Geometry: see drawing. Coordinates: mm, zero at the bounding-box minimum. A direction names the side the tool comes from. Round coordinates to 2 decimals unless told otherwise and drop trailing zeros. Write each loop counter-clockwise with the first axis right and the second up, starting at its lowest first coordinate (ties: lowest second). Pieces come first, ordered by that corner, then holes. Notation, with made-up numbers: M 18.25,73 L 63.25,73 A14 cw 63.25,86 Z; hole C -21,3 d11. An arc over 180 degrees is marked long. Use one line per item in the form item = value. Start each with the question number.
Item 1: Pull-direction query (X, two-part tool) for the marked faces 3, 4 and 5; classes: pulls with the +X half, pulls with the -X half, needs draft (parallel to the pull), parting line crosses it, or undercut.
Item 2: Section query C-C (y = 14.75). Return loops of the section in (x, z), and give its area (3 significant figures).
Item 3: Section query D-D (x = 19.5). Return loops of the section in (y, z), and give its area (3 significant figures).
Item 4: Section query A-A (x = 32.5). Return loops of the section in (y, z), and give its area (3 significant figures).
Item 5: Pin query (flat end, axial travel): pin 1 Ø8 at (y, z) = (13, 27) entering from -X. Return the tip coordinate at first contact, or that it passes through.
Item 6: Reachability of the marked faces 1 and 2 from +Z, -Z, +X, -X, +Y, -Y: full face, straight path, thin tool, end or side. Return the list, or none.
Item 7: Section query B-B (z = 50). Return loops of the section in (x, y).
Item 8: Ray query, probe 1 along Z at (x, y) = (32.5, 29.35); probe 2 along X at (y, z) = (28.6, 50); probe 3 along X at (y, z) = (25, 75.5). Return the intervals inside material, ascending.
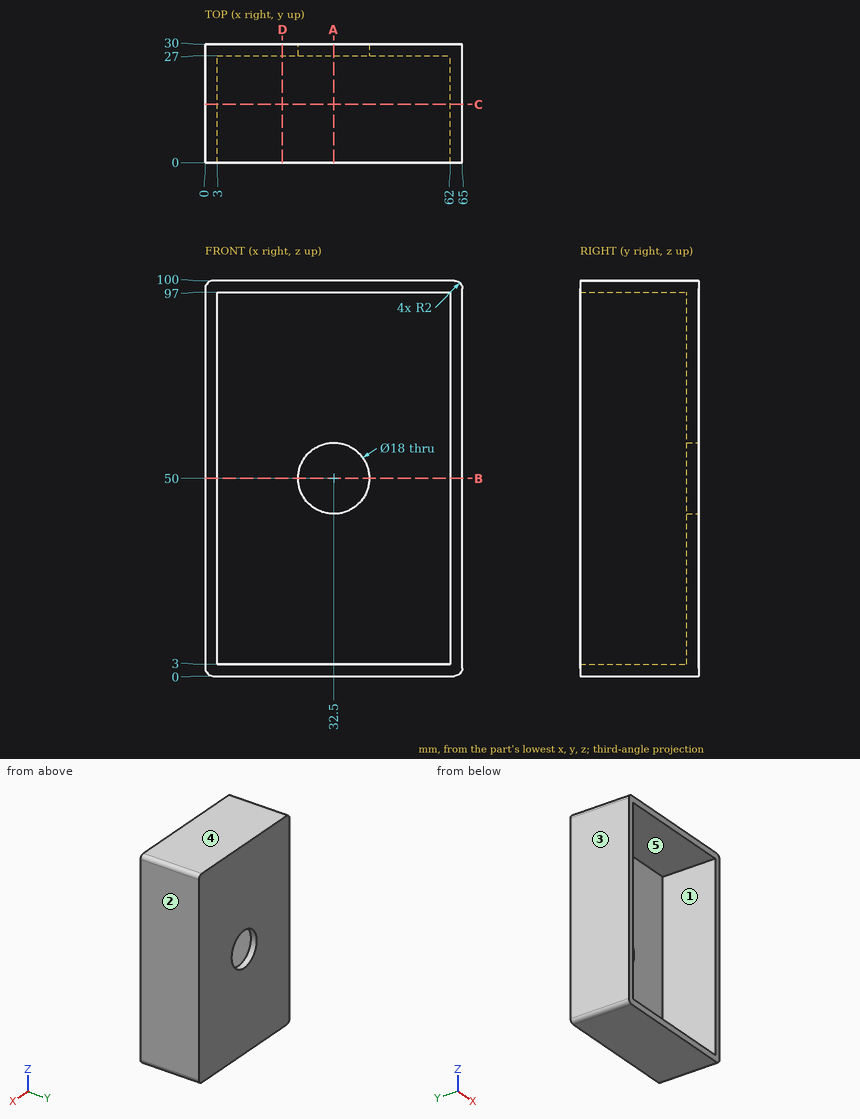
Working result:
q1.face_3 = pulls with the -X half
q1.face_4 = needs draft
q1.face_5 = undercut
q2.outline = M 0,2 A2 ccw 2,0 L 63,0 A2 ccw 65,2 L 65,98 A2 ccw 63,100 L 2,100 A2 ccw 0,98 Z; hole M 3,3 L 62,3 L 62,97 L 3,97 Z
q2.area = 951 mm²
q3.outline = M 0,0 L 30,0 L 30,100 L 0,100 L 0,97 L 27,97 L 27,3 L 0,3 Z
q3.area = 462 mm²
q4.outline = M 0,0 L 30,0 L 30,41 L 27,41 L 27,3 L 0,3 Z; M 0,97 L 27,97 L 27,59 L 30,59 L 30,100 L 0,100 Z
q4.area = 408 mm²
q5.pin_1 = 0
q6.face_1 = -Y
q6.face_2 = +Z, -Z, +X, +Y, -Y
q7.outline = M 0,0 L 3,0 L 3,27 L 23.5,27 L 23.5,30 L 0,30 Z; M 41.5,27 L 62,27 L 62,0 L 65,0 L 65,30 L 41.5,30 Z
q8.probe_1 = 0 to 41, 59 to 100
q8.probe_2 = 0 to 23.5, 41.5 to 65
q8.probe_3 = 0 to 3, 62 to 65
